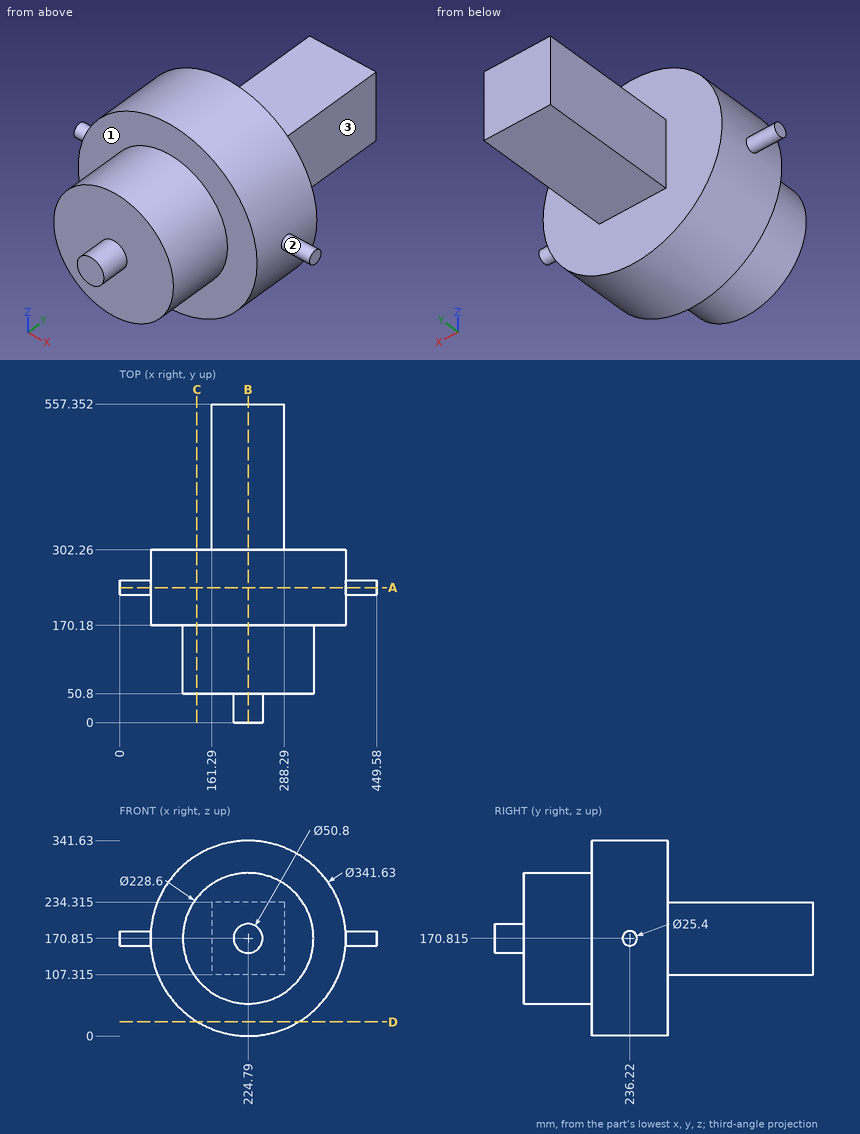
Source: three-view drawing plus pictorial views. Frame: mm from the lowest corner of the part. A direction names the side the tool comes from. Give positions to 0.01 mm unless a question says otherwise; leave off trailing zeros. Write each loop counter-clockwise with the first axis right and the second up, starting at its lowest first coordinate (ties: lowest second). Pieces come first, ordered by that corner, then holes. Notation, with made-up numbers: (-38, 80) - (-31, 80) arc R37 ccw to (-31, 116) - close; hole circle Ø9 at (29, 0). An arc over 180 degrees is marked (long way). Write item = value, one per line. Start each with the question number.
Q1. Cut plane B-B, the plane x = 224.79. Return loops of the section in (y, z) (1 decimal).
Q2. Cut plane D-D, the plane z = 24.5. Return loops of the section in (x, y).
Q3. Pin query (flat end, axial travel): pin 1 Ø1.5 at (x, z) = (185, 56) entering from -Y; pin 2 Ø10 at (x, z) = (177.5, 71) entering from -Y; pin 3 Ø8 at (x, z) = (119, 112.5) entering from +Y. Return the tip coordinate at first contact, or that it passes through.
Q4. Cut plane C-C, the plane x = 135. Return loops of the section in (y, z), then the cut area to 3 significant figures.
Q5. Cut plane A-A, the plane y = 236.22. Return loops of the section in (x, z) (1 decimal).
Q6. Material intervals for probe 1 along Z at (x, y) = (269.5, 488.5) (3 decimals); probe 2 along Y at (x, z) = (329.5, 120); probe 3 along X at (y, z) = (410.5, 207), sorted ascending.
Q7. Reachability of the marked faces 1, 2 and 3 from +Z, -Z, +X, -X, +Y, -Y: full face, straight path, thin tool, end or side. Return the list, or none.
Computed values:
q1.outline = (0, 145.4) - (50.8, 145.4) - (50.8, 56.5) - (170.2, 56.5) - (170.2, 0) - (302.3, 0) - (302.3, 107.3) - (557.4, 107.3) - (557.4, 234.3) - (302.3, 234.3) - (302.3, 341.6) - (170.2, 341.6) - (170.2, 285.1) - (50.8, 285.1) - (50.8, 196.2) - (0, 196.2) - close
q2.outline = (136.64, 170.18) - (312.94, 170.18) - (312.94, 302.26) - (136.64, 302.26) - close
q3.pin_1 = 170.18
q3.pin_2 = 50.8
q3.pin_3 = 302.26
q4.outline = (50.8, 100.09) - (170.18, 100.09) - (170.18, 25.5) - (302.26, 25.5) - (302.26, 316.13) - (170.18, 316.13) - (170.18, 241.54) - (50.8, 241.54) - close
q4.area = 55,300 mm²
q5.outline = (0, 158.1) - (54.4, 158.1) arc R170.8 ccw to (395.1, 158.1) - (449.6, 158.1) - (449.6, 183.5) - (395.1, 183.5) arc R170.8 ccw to (54.4, 183.5) - (0, 183.5) - close
q6.probe_1 = 107.315 to 234.315
q6.probe_2 = 170.18 to 302.26
q6.probe_3 = 161.29 to 288.29
q7.face_1 = -Y
q7.face_2 = +X
q7.face_3 = +Z, -Z, +X, +Y
